Here's how the part is built. I have some questions about the finished solid (model axes, mm). Face numbers are marked on the shaded views. A direction names the side the tool comes from. Give positions to 0.01 mm unless a question says otherwise; leave off trailing zeros. Order: outer loops, then holes, each group sorted by start corner. A loop starts at its lowest first (then second) coordinate and runs counter-clockwise, first axis right, second up.
from build123d import *

# Parameters (mm, degrees)
SKETCH1_R = 0.4


with BuildPart() as part:
    # Sweep1: sweep along a path in Sketch4
    with BuildLine(Plane.XY) as sweep1_path:
        Line((0, 0), (0, 4.5))
        ThreePointArc((0, 4.5), (0.146446609, 4.853553391), (0.5, 5))
        Line((0.5, 5), (11, 5))
        ThreePointArc((11, 5), (11.353553391, 4.853553391), (11.5, 4.5))
        Line((11.5, 4.5), (11.5, 0))
    # Sketch1 → Sweep1 (sweep)
    with BuildSketch(Plane(origin=(0, 0, 0), x_dir=(1, 0, 0), z_dir=(0, 1, 0))):
        Circle(SKETCH1_R)
    sweep(path=sweep1_path.line)


solid = part.part
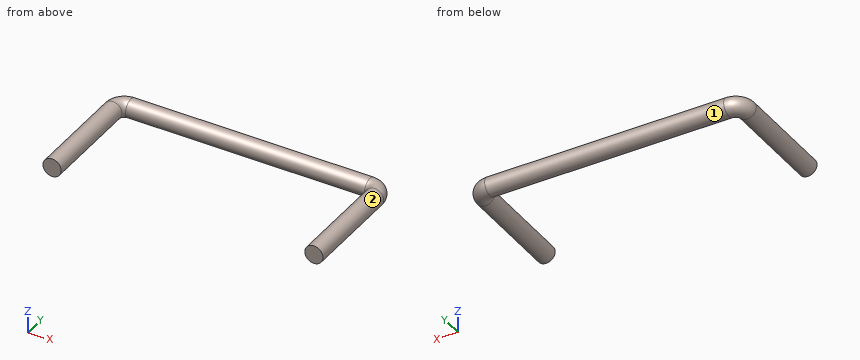
Q1. I need wall thicknesses on L1, parallel to X at y = 3.95, z = -0.05; L2, parallel to X at y = 3.2, z = -0.3; L3, parallel to Z at x = 0.5, y = 4.8. Which ranges of each line are inside material? Lowest first, please.
Filled sheet:
L1: x = -0.4 to 0.4, 11.1 to 11.9
L2: x = -0.26 to 0.26, 11.24 to 11.76
L3: z = -0.35 to 0.35
Q2. If we section it at B-B on z = 0.15: List the corners of the cut face in (x, y) for me.
Filled sheet:
outline: (-0.37, 0) - (0.37, 0) - (0.37, 4.5) arc R0.13 cw to (0.5, 4.63) - (11, 4.63) arc R0.13 cw to (11.13, 4.5) - (11.13, 0) - (11.87, 0) - (11.87, 4.5) arc R0.87 ccw to (11, 5.37) - (0.5, 5.37) arc R0.87 ccw to (-0.37, 4.5) - close
Q3. If we section it at A-A on y = 2.1: List the corners of the cut face in (x, z) for me, plus the area to 3 significant figures.
Filled sheet:
outline: circle Ø0.8 at (0, 0); circle Ø0.8 at (11.5, 0)
area: 1.01 mm2
Q4. If we section it at C-C on x = 1.75: List the corners of the cut face in (y, z) for me.
Filled sheet:
outline: circle Ø0.8 at (5, 0)
Q5. For the marked faces 1 and 2, which set-ups out of +Z, -Z, +X, -X, +Y, -Y let a thin tool reach every point of the face, with its end or its side?
Filled sheet:
face 1: none
face 2: -Y
